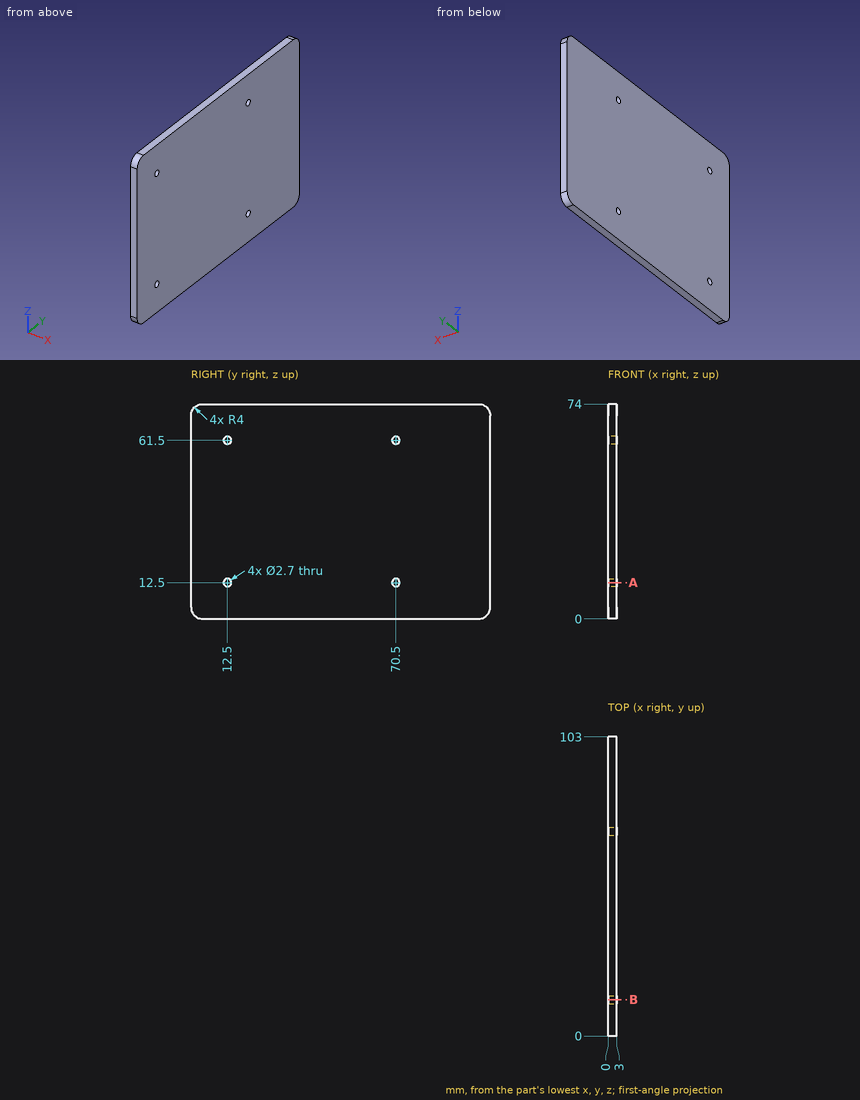
Study the drawing (mm; zero at the part's minimum x, y, z) and answer. Give positions to 0.01 mm unless a question says otherwise; leave off trailing zeros. Order: outer loops, then holes, each group sorted by start corner. A loop starts at its lowest first (then second) coordinate and runs counter-clockwise, first axis right, second up.
1) Consider line 1 along Y through (x, z) = (0.75, 12.5); line 2 along Z through (x, y) = (0.7, 70.5). Determine where each line is inside the solid, lowest interval first.
Reported:
line 1: y = 0 to 11.15, 13.85 to 69.15, 71.85 to 103
line 2: z = 0 to 11.15, 13.85 to 60.15, 62.85 to 74
2) Given P1, Ø4.5, axis at y = 70.5, z = 61.5, coming from the -X side, flat-ended and moving along its own axis, determine where the tip first touches the part or whether it passes through.
Reported:
P1: stops at x = 0
3) Find section B-B on y = 12.5. Write down the section's boundary in (x, z), then the cut area to 3 significant figures.
Reported:
outline: (0, 0) - (3, 0) - (3, 11.15) - (0, 11.15) - close; (0, 13.85) - (3, 13.85) - (3, 60.15) - (0, 60.15) - close; (0, 62.85) - (3, 62.85) - (3, 74) - (0, 74) - close
area: 206 mm2
4) Find section A-A on z = 12.5. Write down the section's boundary in (x, y), then the cut area to 3 significant figures.
Reported:
outline: (0, 0) - (3, 0) - (3, 11.15) - (0, 11.15) - close; (0, 13.85) - (3, 13.85) - (3, 69.15) - (0, 69.15) - close; (0, 71.85) - (3, 71.85) - (3, 103) - (0, 103) - close
area: 293 mm2
